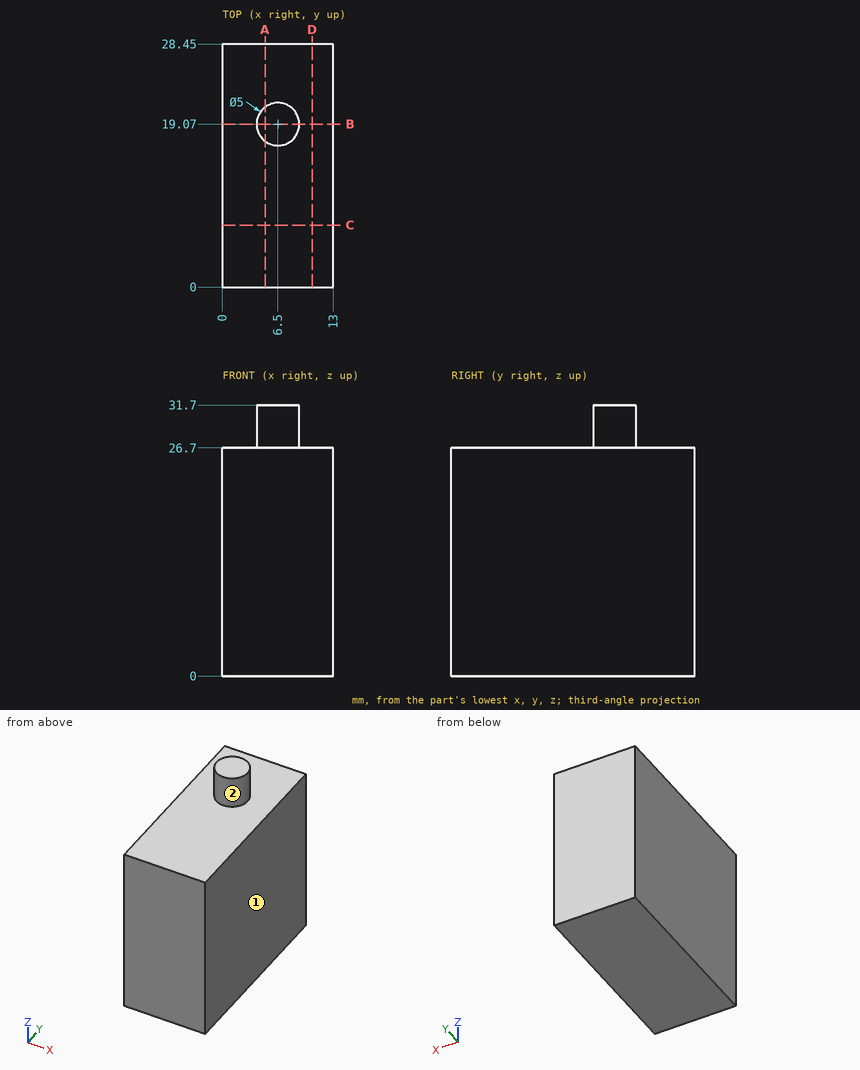
Source: three-view drawing plus pictorial views. Frame: mm from the lowest corner of the part. A direction names the side the tool comes from. Coordinates: 2 decimals unless noted, no trailing zeros. Order: outer loops, then holes, each group sorted by start corner. A loop starts at its lowest first (then second) coordinate and runs counter-clockwise, first axis right, second up.
1) Section D-D (x = 10.5). Return loops of the section in (y, z).
Result sheet:
outline: (0, 0) - (28.45, 0) - (28.45, 26.7) - (0, 26.7) - close
2) Section C-C (y = 7.25). Return loops of the section in (x, z), then the cut area to 3 significant figures.
Result sheet:
outline: (0, 0) - (13, 0) - (13, 26.7) - (0, 26.7) - close
area: 347 mm2
3) Section B-B (y = 19.07). Return loops of the section in (x, z).
Result sheet:
outline: (0, 0) - (13, 0) - (13, 26.7) - (9, 26.7) - (9, 31.7) - (4, 31.7) - (4, 26.7) - (0, 26.7) - close
4) Ray query, probe 1 along Z at (x, y) = (3, 19); probe 2 along X at (y, z) = (19, 30); probe 3 along Y at (x, z) = (8.25, 30). Return the intervals inside material, ascending.
Result sheet:
probe 1: z = 0 to 26.7
probe 2: x = 4 to 9
probe 3: y = 17.28 to 20.86
5) First-contact query: P1, Ø4, axis at x = 9.5, y = 7.5, coming from the +Z side; P2, Ø3, axis at x = 1.5, y = 8.5, coming from the -Z side. Flat tips, straight axial feed; report the tip coordinate or a pass-through.
Result sheet:
P1: stops at z = 26.7
P2: stops at z = 0
6) Set-up query: the marked faces 1 and 2. Return all of +Z, -Z, +X, -X, +Y, -Y with unobstructed straight access to the full face (end or side cutting, diameter ignored); none if empty.
Result sheet:
face 1: +Z, -Z, +X, +Y, -Y
face 2: +Z
7) Section A-A (x = 5). Return loops of the section in (y, z).
Result sheet:
outline: (0, 0) - (28.45, 0) - (28.45, 26.7) - (21.07, 26.7) - (21.07, 31.7) - (17.07, 31.7) - (17.07, 26.7) - (0, 26.7) - close
